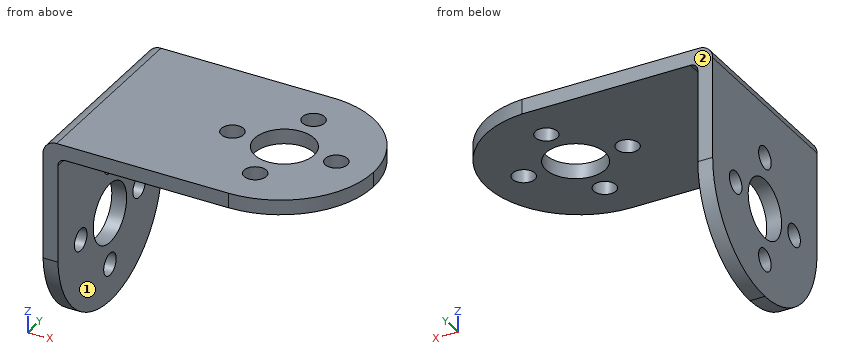
from build123d import *
from OCP.BRepAlgoAPI import BRepAlgoAPI_Cut
from OCP.TopTools import TopTools_ListOfShape

# Parameters (mm, degrees)
SALIENTE_EXTRUIR1_DEPTH     = 25
CROQUIS2_R                  = 4
CROQUIS2_R_2                = 1.5
CORTAR_EXTRUIR1_DEPTH       = 25
CORTAR_EXTRUIR2_START       = -2
CORTAR_EXTRUIR2_OUTLINE_R   = 1.5
CORTAR_EXTRUIR2_OUTLINE_R_2 = 4
CORTAR_EXTRUIR2_DEPTH       = 2


with BuildPart() as part:
    # Croquis1 → Saliente-Extruir1 (new body)
    with BuildSketch(Plane(origin=(0, 0, 0), x_dir=(1, 0, 0), z_dir=(0, 1, 0))):
        with BuildLine():
            Line((0, 1.84), (0, 28))
            Line((0, 28), (2, 28))
            Line((2, 28), (2, 3))
            ThreePointArc((2, 3), (2.292893219, 2.292893219), (3, 2))
            Line((3, 2), (37.5, 2))
            Line((37.5, 2), (37.5, 0))
            Line((37.5, 0), (1.84, 0))
            ThreePointArc((1.84, 0), (0.538923523, 0.538923523), (0, 1.84))
        make_face()
    extrude(amount=SALIENTE_EXTRUIR1_DEPTH)

    # Croquis2 → Cortar-Extruir1 (cut)
    with BuildSketch(Plane.ZY):
        with Locations((-16, 12.49)):
            Circle(CROQUIS2_R)
        with Locations((-23, 12.49)):
            Circle(CROQUIS2_R_2)
        with BuildLine():
            ThreePointArc((-16.197106781, 0), (-24.582469572, 3.897730388), (-28, 12.49))
            Line((-28, 12.49), (-28, 0))
            Line((-28, 0), (-16.197106781, 0))
        make_face()
        with BuildLine():
            Line((-28, 25), (-28, 12.49))
            ThreePointArc((-28, 12.49), (-24.335905833, 21.335905833), (-15.49, 25))
            Line((-15.49, 25), (-28, 25))
        make_face()
        with Locations((-9, 12.49)):
            Circle(CROQUIS2_R_2)
        with Locations((-16, 19.49)):
            Circle(CROQUIS2_R_2)
        with Locations((-16, 5.49)):
            Circle(CROQUIS2_R_2)
    extrude(amount=-CORTAR_EXTRUIR1_DEPTH, mode=Mode.SUBTRACT)


with BuildPart() as cortar_extruir2_tool:
    # Cortar-Extruir2: read off the stored shape, not the designer's step
    # Cortar-Extruir2 outline → Cortar-Extruir2 (new body)
    with BuildSketch(Plane.XY.offset(CORTAR_EXTRUIR2_START)):
        with BuildLine():
            ThreePointArc((25.697106781, 25), (34.082469572, 21.102269612), (37.5, 12.51))
            Line((37.5, 12.51), (37.5, 25))
            Line((37.5, 25), (25.697106781, 25))
        make_face()
        with BuildLine():
            Line((37.5, 0), (37.499996003, 12.500000002))
            ThreePointArc((37.499996003, 12.500000002), (33.832369592, 3.66055934), (24.99, 0))
            Line((24.99, 0), (37.5, 0))
        make_face()
        with Locations((18.5, 12.5)):
            Circle(CORTAR_EXTRUIR2_OUTLINE_R)
        with Locations((25.5, 19.5)):
            Circle(CORTAR_EXTRUIR2_OUTLINE_R)
        with Locations((25.5, 5.5)):
            Circle(CORTAR_EXTRUIR2_OUTLINE_R)
        with Locations((25.5, 12.5)):
            Circle(CORTAR_EXTRUIR2_OUTLINE_R_2)
        with Locations((32.5, 12.5)):
            Circle(CORTAR_EXTRUIR2_OUTLINE_R)
    extrude(amount=CORTAR_EXTRUIR2_DEPTH)


with BuildPart() as part_1:
    add(part.part)

    # Cortar-Extruir2: cut by cortar_extruir2_tool, with a tolerance
    cortar_extruir2_stock = TopTools_ListOfShape()
    cortar_extruir2_stock.Append(part_1.part.wrapped)
    cortar_extruir2_tools = TopTools_ListOfShape()
    cortar_extruir2_tools.Append(cortar_extruir2_tool.part.wrapped)
    cortar_extruir2_cut = BRepAlgoAPI_Cut()
    cortar_extruir2_cut.SetArguments(cortar_extruir2_stock)
    cortar_extruir2_cut.SetTools(cortar_extruir2_tools)
    cortar_extruir2_cut.SetFuzzyValue(0.00001)
    cortar_extruir2_cut.Build()
    add(Compound.cast(cortar_extruir2_cut.Shape()).solids(), mode=Mode.REPLACE)


solid = part_1.part
Read the model definition and answer for the solid it produces. Units are mm, in the model's axes. Face numbers are marked on the shaded views. A direction names the side the tool comes from. Give positions to 0.01 mm unless a question says otherwise; leave off trailing zeros. Loops run counter-clockwise (first coordinate to the right, second up) from the corner with the lowest first, then second, coordinate; pieces in that order, holes last. Notation, with made-up numbers: (6, -24.75) -> (10, -24.75) arc R16 ccw to (10, 5.25) -> close; hole circle Ø3 at (86, 82.25). An arc over 180 degrees is marked (long way). Use a Markdown table: item, result.
Q1. Section A-A, the plane z = -9 is taken. Determine the outline of the cut face in (x, y).
Solved:
| item | result |
|---|---|
| outline | (0, 0) -> (2, 0) -> (2, 10.99) -> (0, 10.99) -> close; (0, 13.99) -> (2, 13.99) -> (2, 25) -> (0, 25) -> close |
Q2. Section D-D, the plane y = 3 is taken. Determine the outline of the cut face in (x, z).
Solved:
| item | result |
|---|---|
| outline | (0, -23.64) -> (2, -23.64) -> (2, -3) arc R1 cw to (3, -2) -> (33.12, -2) -> (33.12, 0) -> (1.84, 0) arc R1.84 ccw to (0, -1.84) -> close |
Q3. Section C-C, the plane x = 19.5 is taken. Determine the outline of the cut face in (y, z).
Solved:
| item | result |
|---|---|
| outline | (0, -2) -> (11.38, -2) -> (11.38, 0) -> (0, 0) -> close; (13.62, -2) -> (25, -2) -> (25, 0) -> (13.62, 0) -> close |
Q4. A tool of negligible diameter and unlimited length cuts with its end or side. For the marked faces 1 and 2, from which of +Z, -Z, +X, -X, +Y, -Y can it reach the whole face along a straight path? Write none if from no direction.
Solved:
| item | result |
|---|---|
| face 1 | -Z, +X, +Y, -Y |
| face 2 | +Z, -Z, +X, -X, +Y |
Q5. Each of these flat-tipped pins is pushed along its axis until it touches: pin 1 (6 mm diameter, centred on x = 7, y = 9.5, fed in from -Z); pin 2 (10 mm diameter, centred on y = 14, z = -17, fed in from +X); pin 3 (3.5 mm diameter, centred on x = 32.5, y = 12.5, fed in from +Z). Where does it stop, or does it pass through?
Solved:
| item | result |
|---|---|
| pin 1 | stops at z = -2 |
| pin 2 | stops at x = 2 |
| pin 3 | stops at z = 0 |
Q6. Find the intervals of material crossed by line 1 along Y through (x, z) = (1.2, -9); line 2 along Y through (x, z) = (25.5, -1.3); line 3 along X through (y, z) = (5, -12.25), in increasing order.
Solved:
| item | result |
|---|---|
| line 1 | y = 0 to 10.99, 13.99 to 25 |
| line 2 | y = 0.01 to 4, 7 to 8.5, 16.5 to 18, 21 to 25 |
| line 3 | x = 0 to 2 |
Q7. Section B-B, the plane x = 26.5 is taken. Determine the outline of the cut face in (y, z), then the cut area to 3 significant figures.
Solved:
| item | result |
|---|---|
| outline | (0.09, -2) -> (4.38, -2) -> (4.38, 0) -> (0.09, 0) -> close; (6.62, -2) -> (8.63, -2) -> (8.63, 0) -> (6.62, 0) -> close; (16.37, -2) -> (18.38, -2) -> (18.38, 0) -> (16.37, 0) -> close; (20.62, -2) -> (24.93, -2) -> (24.93, 0) -> (20.62, 0) -> close |
| area | 25.2 mm^2 |
